Could you check a few things on this model? Use its own coordinates, in mm. Face numbers are marked on the shaded views. Round coordinates to 2 decimals unless told otherwise and drop trailing zeros. Order: outer loops, then holes, each group sorted by start corner. A loop starts at its lowest first (then second) coordinate and runs counter-clockwise, first axis right, second up. Notation, with made-up numbers: (-10, 50) - (13, 50) arc R27 ccw to (13, 69) - close; hole circle Ø7 at (77, -1.75). An arc over 180 degrees is marked (long way). Use one line per item in the form item = value.
from build123d import *

# Parameters (mm, degrees)
SKETCH3_W           = 8
SKETCH3_H           = 2
BOSS_EXTRUDE2_DEPTH = 31.75
SKETCH4_R           = 2.1
CUT_EXTRUDE1_DEPTH  = 3


with BuildPart() as part:
    # Sketch3 → Boss-Extrude2 (new body)
    with BuildSketch(Plane(origin=(0, 0, 0), x_dir=(1, 0, 0), z_dir=(0, 1, 0))):
        with Locations((2.282032354, 3.507256135)):
            Rectangle(SKETCH3_W, SKETCH3_H)
    extrude(amount=BOSS_EXTRUDE2_DEPTH)

    # Sketch4 → Cut-Extrude1 (cut, through all)
    with BuildSketch(Plane.XY.offset(-2.507256135)):
        with Locations((2.282032354, 7.875)):
            Circle(SKETCH4_R)
        with Locations((2.282032354, 23.875)):
            Circle(SKETCH4_R)
    extrude(amount=-CUT_EXTRUDE1_DEPTH, mode=Mode.SUBTRACT)


solid = part.part
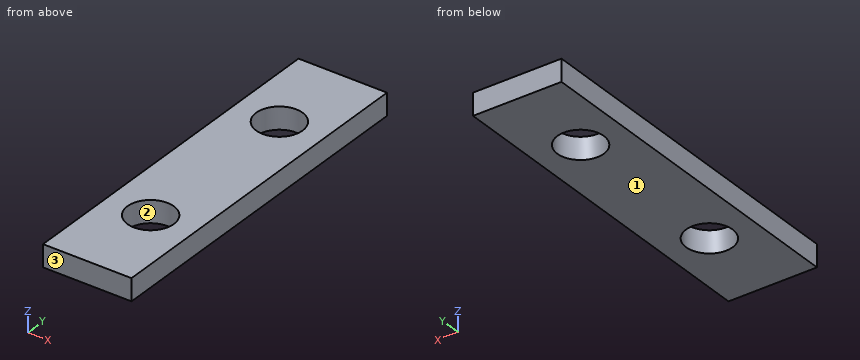
Item 1: Imagine slicing it at C-C on x = 0.5. Please give me the cut outline in (y, z), plus the area to 3 significant figures.
Found:
outline = (0, -4.51) - (6.76, -4.51) - (6.76, -2.51) - (0, -2.51) - close; (8.99, -4.51) - (22.76, -4.51) - (22.76, -2.51) - (8.99, -2.51) - close; (24.99, -4.51) - (31.75, -4.51) - (31.75, -2.51) - (24.99, -2.51) - close
area = 54.6 mm2
Item 2: Imagine slicing it at D-D on z = -3.2. Please give me the cut outline in (x, y) (3 decimals), plus the area to 3 significant figures.
Found:
outline = (-1.718, 0) - (6.282, 0) - (6.282, 31.75) - (-1.718, 31.75) - close; hole circle Ø4.2 at (2.282, 7.875); hole circle Ø4.2 at (2.282, 23.875)
area = 226 mm2
Item 3: If we mould it in two halves opening along Y, with no side actions, what happens to the marked faces 1, 2 and 3? For each: released by +Y, released by -Y, zero draft, split by the parting line, or undercut.
Found:
face_1 = zero draft
face_2 = undercut
face_3 = released by -Y
Item 4: Imagine slicing it at A-A on x = 3. Please give me the cut outline in (y, z), plus the area to 3 significant figures.
Found:
outline = (0, -4.51) - (5.9, -4.51) - (5.9, -2.51) - (0, -2.51) - close; (9.85, -4.51) - (21.9, -4.51) - (21.9, -2.51) - (9.85, -2.51) - close; (25.85, -4.51) - (31.75, -4.51) - (31.75, -2.51) - (25.85, -2.51) - close
area = 47.7 mm2
Item 5: Imagine slicing it at B-B on y = 23.5. Please give me the cut outline in (x, z), plus the area to 4 significant figures.
Found:
outline = (-1.72, -4.51) - (0.22, -4.51) - (0.22, -2.51) - (-1.72, -2.51) - close; (4.35, -4.51) - (6.28, -4.51) - (6.28, -2.51) - (4.35, -2.51) - close
area = 7.735 mm2
Item 6: I need wall thicknesses on L1, parallel to Y at x = 2, z = -4.2; L2, parallel to Y at x = 3, z = -3.65; L3, parallel to X at y = 22, z = -2.65. Which ranges of each line are inside material? Lowest first, please.
Found:
L1 = 0 to 5.79, 9.96 to 21.79, 25.96 to 31.75
L2 = 0 to 5.9, 9.85 to 21.9, 25.85 to 31.75
L3 = -1.72 to 1.34, 3.23 to 6.28
